Check sheet for the modelled part. Datum: model origin and axes. Units: mm. Face numbers are marked on the shaded views. A direction names the side the tool comes from. Round coordinates to 2 decimals unless told otherwise and drop trailing zeros. Order: outer loops, then holes, each group sorted by start corner. A loop starts at its lowest first (then second) coordinate and runs counter-clockwise, first axis right, second up.
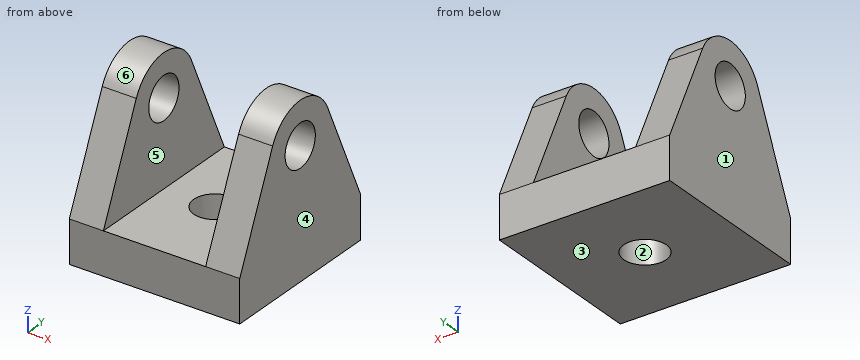
Autodesk Inventor part; units mm, degrees
ref_plane "YZ Plane" through (0, 0, 0) normal (1, 0, 0) x (0, 1, 0)
ref_plane "XZ Plane" through (0, 0, 0) normal (0, 1, 0) x (-1, 0, 0)
ref_plane "XY Plane" through (0, 0, 0) normal (0, 0, 1) x (1, 0, 0)
sketch "Sketch1" plane through (0, 0, 0) normal (0, 0, 1) x (1, 0, 0)
  line L0 (0, 0) -> (25.4, 0)
  line L1 (25.4, 0) -> (25.4, 25.4)
  line L2 (25.4, 25.4) -> (0, 25.4)
  line L3 (0, 25.4) -> (0, 0)
  dimension "d0" = 25.4
  dimension "d1" = 25.4
extrude "Extrusion1" add sketch "Sketch1" along normal blind 25.4
sketch "Sketch2" plane through (25.4, 0, 0) normal (1, 0, 0) x (0, 0, -1)
  line L0 (0, 0) -> (0, 25.4)
  line L1 (0, 25.4) -> (-25.4, 25.4)
  line L2 (-25.4, 0) -> (-25.4, 25.4)
  line L3 (0, 0) -> (-25.4, 0)
  circle A0 centre (-19.05, 12.7) radius 6.35
  line L4 (-21.6626, 18.4876) -> (-6.35, 25.4)
  line L5 (-21.6626, 6.9124) -> (-6.35, 0)
  line L6 (0, 12.7) -> (-19.05, 12.7) construction
  dimension "d4" = 12.7
  dimension "d5" = 6.35
extrude "Extrusion2" cut sketch "Sketch2" against normal through all contours L3 L2 A0 L5 | L4 A0 L2 L1
sketch "Sketch3" plane through (25.4, 0, 0) normal (1, 0, 0) x (0, 0, -1)
  arc A0 (-21.6626, 18.4876) -> (-21.6626, 6.9124) centre (-19.05, 12.7) ccw
hole "Hole1" at (25.4, 12.7, 19.05) direction (-1, 0, 0) diameter 6.35 end through all
sketch "Sketch4" plane through (0, 25.4, 0) normal (0, 1, 0) x (1, 0, 0)
  line L0 (0, -6.35) -> (25.4, -6.35)
  line L1 (25.4, 0) -> (25.4, -6.35)
  line L2 (0, 0) -> (0, -6.35)
  line L3 (25.4, -25.4) -> (0, -25.4)
  line L4 (5.08, -6.35) -> (20.32, -6.35)
  line L5 (20.32, -6.35) -> (20.32, -25.4)
  line L6 (20.32, -25.4) -> (5.08, -25.4)
  line L7 (5.08, -25.4) -> (5.08, -6.35)
  dimension "d15" = 5.08
  dimension "d16" = 5.08
extrude "Extrusion3" cut sketch "Sketch4" against normal through all
sketch "Sketch5" plane through (0, 0, 0) normal (0, 0, -1) x (-1, 0, 0)
  line L0 (-25.4, 25.4) -> (0, 0) construction
  circle A0 centre (-12.7, 12.7) radius 3.175
  dimension "d19" = 6.35
extrude "Extrusion4" cut sketch "Sketch5" against normal through all
equation "\"d16\" = d15"
properties part number "Joint" material "Aluminum 6061"
Item 1: Release check for a two-part mould opening along X. For the marked faces 1, 2, 3 and 4 record: released by +X, released by -X, zero draft, split by the parting line, or undercut.
Answer:
face 1: released by -X
face 2: undercut
face 3: zero draft
face 4: released by +X
Item 2: Sectioned sample at C-C (x = 12.7). Record the cut outline in (y, z) (3 decimals), and give its area (3 significant figures).
Answer:
outline: (0, 0) - (9.525, 0) - (9.525, 6.35) - (0, 6.35) - close; (15.875, 0) - (25.4, 0) - (25.4, 6.35) - (15.875, 6.35) - close
area: 121 mm2
Item 3: Sectioned sample at D-D (z = 7.25). Record the cut outline in (x, y), and give its area (3 significant figures).
Answer:
outline: (0, 0.41) - (5.08, 0.41) - (5.08, 24.99) - (0, 24.99) - close; (20.32, 0.41) - (25.4, 0.41) - (25.4, 24.99) - (20.32, 24.99) - close
area: 250 mm2
Item 4: Access from +Z, -Z, +X, -X, +Y, -Y to the whole of each face (thin tool, end or side, straight path). Record for the marked faces 5 and 6.
Answer:
face 5: +Z, +Y, -Y
face 6: +Z, +X, -X
Item 5: Go/stop test with flat-tipped pins: P1, Ø5.5, axis at y = 12.7, z = 19.05, coming from the -X side; P2, Ø7.5, axis at x = 13, y = 15.5, coming from the +Z side. Record where each tip stops, or that it passes through.
Answer:
P1: passes through
P2: stops at z = 6.35
Item 6: Sectioned sample at B-B (z = 19.05). Record the cut outline in (x, y) (3 decimals), and give its area (3 significant figures).
Answer:
outline: (0, 5.733) - (5.08, 5.733) - (5.08, 9.525) - (0, 9.525) - close; (0, 15.875) - (5.08, 15.875) - (5.08, 19.667) - (0, 19.667) - close; (20.32, 5.733) - (25.4, 5.733) - (25.4, 9.525) - (20.32, 9.525) - close; (20.32, 15.875) - (25.4, 15.875) - (25.4, 19.667) - (20.32, 19.667) - close
area: 77.1 mm2
Item 7: Sectioned sample at A-A (y = 12.7). Record the cut outline in (x, z) (3 decimals).
Answer:
outline: (0, 0) - (9.525, 0) - (9.525, 6.35) - (5.08, 6.35) - (5.08, 15.875) - (0, 15.875) - close; (0, 22.225) - (5.08, 22.225) - (5.08, 25.4) - (0, 25.4) - close; (15.875, 0) - (25.4, 0) - (25.4, 15.875) - (20.32, 15.875) - (20.32, 6.35) - (15.875, 6.35) - close; (20.32, 22.225) - (25.4, 22.225) - (25.4, 25.4) - (20.32, 25.4) - close
Item 8: Scan lines: line 1 along Z through (x, y) = (2.4, 12.7) (3 decimals); line 2 along X through (y, z) = (10.75, 8); line 3 along Z through (x, y) = (14.25, 24.25). Record each from-to range of solid material in increasing order.
Answer:
line 1: z = 0 to 15.875, 22.225 to 25.4
line 2: x = 0 to 5.08, 20.32 to 25.4
line 3: z = 0 to 6.35
